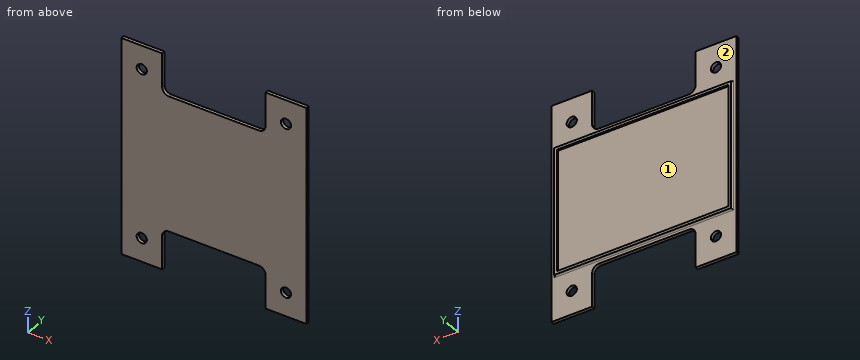
```python
from build123d import *

# Parameters (mm, degrees)
SKETCH1_W                    = 172.72
SKETCH1_H                    = 203.2
BOSS_EXTRUDE1_DEPTH          = 3.175
SKETCH2_W                    = 96.52
SKETCH2_H                    = 38.1
CUT_EXTRUDE1_DEPTH           = 134.381746221
FILLET1_R                    = 6.35
SKETCH6_W                    = 165.1
SKETCH6_H                    = 119.38
SKETCH6_W_2                  = 160.02
SKETCH6_H_2                  = 114.3
BOSS_EXTRUDE2_DEPTH          = 1.7145
FILLET2_R                    = 1.27
F_3_8_0_375_DIAMETER_HOLE1_D = 9.525
MIRROR5_COPY_1_D             = 9.525


with BuildPart() as part:
    # Sketch1 → Boss-Extrude1 (new body)
    with BuildSketch(Plane(origin=(0, 0, 0), x_dir=(1, 0, 0), z_dir=(0, 1, 0))):
        Rectangle(SKETCH1_W, SKETCH1_H)
    extrude(amount=BOSS_EXTRUDE1_DEPTH)

    # Sketch2 → Cut-Extrude1 (cut, through all)
    with BuildSketch(Plane(origin=(0, 3.175, 0), x_dir=(1, 0, 0), z_dir=(0, 1, 0))):
        with Locations((0, 82.55)):
            Rectangle(SKETCH2_W, SKETCH2_H)
        with Locations((0, -82.55)):
            Rectangle(SKETCH2_W, SKETCH2_H)
    extrude(amount=-CUT_EXTRUDE1_DEPTH, mode=Mode.SUBTRACT)

    # Fillet1
    fillet1_edges = [part.edges().sort_by_distance(p)[0] for p in [
        (-48.26, 1.5875, -63.5),
        (48.26, 1.5875, -63.5),
        (-48.26, 1.5875, 63.5),
        (48.26, 1.5875, 63.5),
    ]]
    fillet(fillet1_edges, radius=FILLET1_R)

    # Sketch6 → Boss-Extrude2 (add)
    with BuildSketch(Plane(origin=(0, 3.175, 0), x_dir=(1, 0, 0), z_dir=(0, 1, 0))):
        Rectangle(SKETCH6_W, SKETCH6_H)
        Rectangle(SKETCH6_W_2, SKETCH6_H_2, mode=Mode.SUBTRACT)
    extrude(amount=BOSS_EXTRUDE2_DEPTH)

    # Fillet2
    fillet2_edges = [part.edges().sort_by_distance(p)[0] for p in [
        (82.55, 3.175, 0),
        (0, 3.175, -59.69),
        (-82.55, 3.175, 0),
        (0, 3.175, 59.69),
    ]]
    fillet(fillet2_edges, radius=FILLET2_R)

    # 3/8 (0.375) Diameter Hole1 (through all)
    with Locations(Plane(origin=(0, 3.175, 0), x_dir=(1, 0, 0), z_dir=(0, 1, 0))):
        with Locations((-67.31, -79.375)):
            f_3_8_0_375_diameter_hole1 = Hole(F_3_8_0_375_DIAMETER_HOLE1_D / 2)

    # Mirror4: 3/8 (0.375) Diameter Hole1 across plane
    add(f_3_8_0_375_diameter_hole1.mirror(Plane.XY), mode=Mode.SUBTRACT)

    # Mirror5: 3/8 (0.375) Diameter Hole1 across plane
    add(f_3_8_0_375_diameter_hole1.mirror(Plane(origin=(0, 0, 0), x_dir=(0, 0, 1), z_dir=(1, 0, 0))), mode=Mode.SUBTRACT)

    # Mirror5 copy 1 (through all)
    with Locations(Plane(origin=(0, 3.175, 0), x_dir=(-1, 0, 0), z_dir=(0, 1, 0))):
        with Locations((-67.31, -79.375)):
            Hole(MIRROR5_COPY_1_D / 2)


solid = part.part
```
Source: CAD feature listing. Evaluate the final solid. Frame: model axes, mm. Face numbers are marked on the shaded views. Give positions to 0.01 mm unless a question says otherwise; leave off trailing zeros. Use a Markdown table: item, result.
Q1. Pull-direction query (X, two-part tool) for the marked faces 1 and 2; classes: +X half, -X half, draft (parallel to the pull), parting line (faces both ways), or undercut.
A:
| item | result |
|---|---|
| face 1 | undercut |
| face 2 | draft |
Q2. Section A-A (x = 67.31). State how many separate pieces and enclosed holes the cut face has, and give its area (3 significant figures).
A:
| item | result |
|---|---|
| separate pieces | 3 |
| enclosed holes | 0 |
| area | 594 mm^2 |
Q3. First-contact query: P1, Ø1, axis at x = -10, y = 1, coming from the -Z side; P2, Ø4, axis at x = 36.5, z = 35, coming from the +Y side (3 decimals); P3, Ø0.5, axis at x = -18, y = 4.5, coming from the -Z side. Flat tips, straight axial feed; report the tip coordinate or a pass-through.
A:
| item | result |
|---|---|
| P1 | z = -63.5 |
| P2 | y = 3.175 |
| P3 | z = -59.71 |
Q4. Material intervals for line 1 (Z direction, x = 67.31, y = 2.25); line 2 (X direction, y = 0.4, z = 72); line 3 (Z direction, x = -64.5, y = 3.1), sorted ascending. Write a range as [from, to].
A:
| item | result |
|---|---|
| line 1 | [-101.6, -84.14], [-74.61, 74.61], [84.14, 101.6] |
| line 2 | [-86.36, -48.26], [48.26, 86.36] |
| line 3 | [-101.6, -83.22], [-75.53, 75.53], [83.22, 101.6] |
